Autodesk Inventor part; units mm, degrees
ref_plane "Plano de trabajo1" through (-8.6166, 33.1799, 0) normal (-1, 0, 0) x (0, 0, -1)
ref_plane "Plano de trabajo2" through (0, 0, -307.9) normal (0, 0, 1) x (1, 0, 0)
ref_plane "YZ Plane" through (0, 0, 0) normal (1, 0, 0) x (0, 1, 0)
sketch "Boceto3" plane through (0, 0, 0) normal (0, 0, 1) x (1, 0, 0)
  line L0 (-13.5546, 31.7799) -> (-18.7766, 31.7799)
  line L1 (-12.1166, 33.1799) -> (-12.1166, 30.6799)
  line L2 (-12.1166, 30.6799) -> (-12.8266, 30.6799)
  line L3 (-12.8266, 30.6799) -> (-13.5546, 31.7799)
  arc A0 (-18.7766, 31.7799) -> (-21.5166, 29.0399) centre (-18.7766, 29.0399) ccw
  line L4 (-12.1166, 33.1799) -> (-8.6166, 33.1799)
  line L5 (-21.5166, 29.0399) -> (-21.5166, 26.2799)
  arc A1 (-8.6166, 33.1799) -> (-8.6166, 26.2799) centre (6.7872, 29.7299) ccw
  line L6 (-21.5166, 26.2799) -> (-21.0166, 26.2799)
  line L7 (-8.6166, 26.2799) -> (-9.1166, 26.2799)
  line L8 (-8.6166, 38.7215) -> (-8.6166, 22.0906) construction
  arc A2 (-9.1166, 26.2799) -> (-21.0166, 26.2799) centre (-15.0666, 20.0463) ccw
  dimension "d218" = 2.5
  dimension "d219" = 0.71
  dimension "d221" = 33.5
  dimension "d223" = 2.74
  dimension "d281" = 3.5
  dimension "d288" = 2.76
  dimension "d291" = 0.5
  dimension "d292" = 0.5
  dimension "d301" = 5.2219
extrude "Extrusión4" add sketch "Boceto3" against normal blind 615.8
ref_plane "Plano de trabajo1" through (-8.6166, 33.1799, 0) normal (-1, 0, 0) x (0, 0, -1)
ref_plane "Plano de trabajo2" through (0, 0, -307.9) normal (0, 0, 1) x (1, 0, 0)
sketch "Boceto5" plane through (-8.6166, 33.1799, 0) normal (-1, 0, 0) x (0, 0, -1)
  line L0 (0, 0) -> (0, 6.9)
  line L1 (0, 0) -> (615.8, 0)
  line L2 (6.9, 0) -> (0, 0)
  line L3 (0, 0) -> (0, 6.9)
  line L4 (0, 6.9) -> (615.8, 6.9)
  line L5 (0, 6.9) -> (6.9, 0)
  point P0 (0, 0)
  dimension "d300" = 45
extrude "Extrusión6" cut sketch "Boceto5" along normal through all
mirror "Simetría3" about plane through (0, 0, -307.9) normal (0, 0, 1) of "Extrusión6"
properties part number "SP40-02 JUNTA INT CRISTAL 761 mm" material "Caucho"
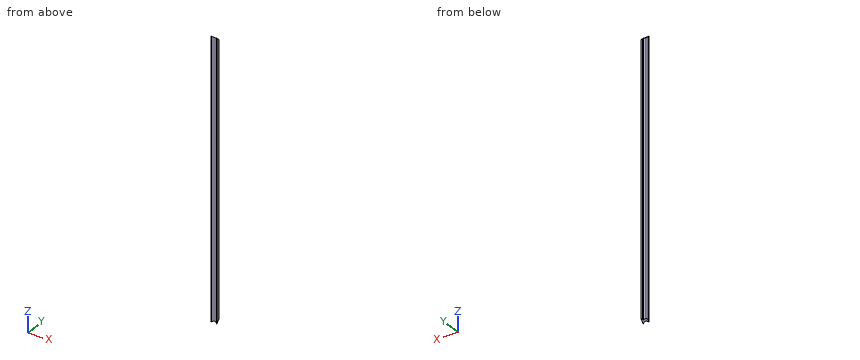
The listing builds one solid part. Answer for the finished solid, in the listing's coordinates (mm). Round coordinates to 2 decimals unless told otherwise and drop trailing zeros. Write each loop counter-clockwise with the first axis right and the second up, starting at its lowest first coordinate (ties: lowest second). Pieces come first, ordered by that corner, then holes. Notation, with made-up numbers: (5.5, -18.75) -> (36.5, -18.75) arc R16 cw to (36.5, -14.75) -> close; hole circle Ø11 at (25, 27). An arc over 180 degrees is marked (long way). Answer as a JSON object with one key per item and string values. Group by question number.
Q1. Each of these flat-tipped pins is pushed along its axis until it touches: pin 1 Ø1 at (y, z) = (31.5, -501.5) entering from -X; pin 2 Ø3 at (y, z) = (32, -206) entering from -X; pin 3 Ø0.6 at (x, z) = (-12.5, -192.5) entering from +Y. Where does it stop, or does it pass through?
Q2. Section A-A (z = -515.5) is taken. Write down the section's boundary in (x, y), plus the area to 3 significant figures.
Q3. Straight lines are drawn through the part: line 1 along X through (y, z) = (30.75, -549.5); line 2 along Z through (x, y) = (-17.5, 30.75); line 3 along Y through (x, z) = (-15.25, -384.5). For each, find the intervals that lie inside material, in ascending order.
Q4. Section B-B (x = -16) is taken. Write down the section's boundary in (y, z), plus the area to 3 significant figures.
Check values:
{
 "1": {"pin 1": "x = -20.69", "pin 2": "x = -21.1", "pin 3": "y = 30.68"},
 "2": {"outline": "(-21.52, 26.28) -> (-21.02, 26.28) arc R8.62 cw to (-9.12, 26.28) -> (-8.62, 26.28) arc R15.79 cw to (-8.62, 33.18) -> (-12.12, 33.18) -> (-12.12, 30.68) -> (-12.83, 30.68) -> (-13.55, 31.78) -> (-18.78, 31.78) arc R2.74 ccw to (-21.52, 29.04) -> close", "area": "51.8 mm^2"},
 "3": {"line 1": "-20.92 to -12.87, -12.12 to -8.97", "line 2": "-611.33 to -4.47", "line 3": "28.66 to 31.78"},
 "4": {"outline": "(28.61, -613.47) -> (31.78, -610.3) -> (31.78, -5.5) -> (28.61, -2.33) -> close", "area": "1,930 mm^2"}
}
